```python
from build123d import *

# Parameters (mm, degrees)
EXTRUDE_DEPTH               = 6
EXTRUDE001_DEPTH            = 6
THICKNESS_T                 = 1
BOX002_W                    = 20
BOX002_H                    = 2
BOX002_DEPTH                = 43
BOX_W                       = 5
BOX_H                       = 20
BOX_DEPTH                   = 5
BOX001_W                    = 20
BOX001_H                    = 4
BOX001_DEPTH                = 45
CYLINDER001_W               = 52
CYLINDER001_H               = 50
CYLINDER001_ANGLE           = 60
CYLINDER001_PLACEMENT_ANGLE = 60
CYLINDER_W                  = 54
CYLINDER_H                  = 50
CYLINDER_ANGLE              = 60
CYLINDER_PLACEMENT_ANGLE    = 60


with BuildPart() as extrude_body:
    with BuildSketch(Plane(origin=(8.5, 45, 6), x_dir=(1, 0, 0), z_dir=(0, 1, 0))):
        with BuildLine():
            Line((5, 4), (-5, 4))
            Line((-5, 4), (-5, -3.142136))
            ThreePointArc((-5, -3.142136), (-2.53653, -3.783978), (0, -4))
            ThreePointArc((0, -4), (2.53653, -3.783978), (5, -3.142136))
            Line((5, -3.142136), (5, 4))
        make_face()
    extrude(amount=EXTRUDE_DEPTH)


with BuildPart() as extrude001:
    with BuildSketch(Plane(origin=(8.5, 45, 6), x_dir=(1, 0, 0), z_dir=(0, 1, 0))):
        with BuildLine():
            Line((5, 4), (-5, 4))
            Line((-5, 4), (-5, -3.142136))
            ThreePointArc((-5, -3.142136), (-2.53653, -3.783978), (0, -4))
            ThreePointArc((0, -4), (2.53653, -3.783978), (5, -3.142136))
            Line((5, -3.142136), (5, 4))
        make_face()
    extrude(amount=EXTRUDE001_DEPTH)


with BuildPart() as fusion002:
    # Thickness base: copy of Extrude body
    add(extrude_body.part)

    # Thickness
    thickness_openings = [fusion002.faces().sort_by_distance(p)[0] for p in [
        (8.5, 51, 5.862901),
    ]]
    offset(amount=THICKNESS_T, openings=thickness_openings)

    # Fusion002: union Extrude body, Extrude001
    add(extrude_body.part)
    add(extrude001.part)


with BuildPart() as fusion002_1:
    # Fusion002 placement: moved
    add(fusion002.part.moved(Location((0, -3, 20))))


with BuildPart() as slot:
    # Box002 → Box002 (new body)
    with BuildSketch(Plane(origin=(2, 44, 3.5), x_dir=(1, 0, 0), z_dir=(0, 0, 1))):
        with Locations((10, 1)):
            Rectangle(BOX002_W, BOX002_H)
    extrude(amount=BOX002_DEPTH)


with BuildPart() as pin_opening:
    # Box → Box (new body)
    with BuildSketch(Plane(origin=(7, 42, 5), x_dir=(1, 0, 0), z_dir=(0, 0, 1))):
        with Locations((2.5, 10)):
            Rectangle(BOX_W, BOX_H)
    extrude(amount=BOX_DEPTH)


with BuildPart() as latch:
    # Box001 → Box001 (new body)
    with BuildSketch(Plane(origin=(0, 44, 2.5), x_dir=(1, 0, 0), z_dir=(0, 0, 1))):
        with Locations((10, 2)):
            Rectangle(BOX001_W, BOX001_H)
    extrude(amount=BOX001_DEPTH)


with BuildPart() as bottle_wall001:
    # Cylinder001 → Cylinder001 (revolve)
    with BuildSketch(Plane.XZ):
        with Locations((26, 25)):
            Rectangle(CYLINDER001_W, CYLINDER001_H)
    revolve(axis=Axis((0, 0, 0), (0, 0, 1)), revolution_arc=CYLINDER001_ANGLE)


with BuildPart() as bottle_wall001_1:
    # Cylinder001 placement: moved
    add(bottle_wall001.part.moved(Location((8.5, -7, 0))).rotate(Axis((8.5, -7, 0), (0, 0, 1)), CYLINDER001_PLACEMENT_ANGLE))


with BuildPart() as cut003:
    # Cylinder → Cylinder (revolve)
    with BuildSketch(Plane.XZ):
        with Locations((27, 25)):
            Rectangle(CYLINDER_W, CYLINDER_H)
    revolve(axis=Axis((0, 0, 0), (0, 0, 1)), revolution_arc=CYLINDER_ANGLE)


with BuildPart() as cut003_1:
    # Cylinder placement: moved
    add(cut003.part.moved(Location((8.5, -7, 0))).rotate(Axis((8.5, -7, 0), (0, 0, 1)), CYLINDER_PLACEMENT_ANGLE))

    # Cut: cut bottle_wall001
    add(bottle_wall001_1.part, mode=Mode.SUBTRACT)


with BuildPart() as cut003_2:
    # Cut placement: moved
    add(cut003_1.part.moved(Location((0, -2, 0))))

    # Fusion: union latch
    add(latch.part)

    # Fusion001: union latch
    add(latch.part)

    # Cut001: cut pin_opening
    add(pin_opening.part, mode=Mode.SUBTRACT)

    # Cut002: cut slot
    add(slot.part, mode=Mode.SUBTRACT)

    # Cut003: cut Fusion002
    add(fusion002_1.part, mode=Mode.SUBTRACT)


solid = cut003_2.part
```
Build history of the part. All positions in model axes, mm. A direction names the side the tool comes from. Round coordinates to 2 decimals unless told otherwise and drop trailing zeros. Loops run counter-clockwise (first coordinate to the right, second up) from the corner with the lowest first, then second, coordinate; pieces in that order, holes last.
Item 1: Pin check, flat tips, straight feed: P1, Ø3, axis at y = 46, z = 30, coming from the -X side; P2, Ø8, axis at x = -7, z = 41.5, coming from the -Y side; P3, Ø5, axis at x = -9.5, z = 28.5, coming from the -Y side. Stop position of each tip, or through.
Item 2: Two-plate mould, pull along Y, no slides. Class faces 5 (the face through (11, 45, 46.5)), 6 (the face through (-18, 36.9, 25.4)), 7 (the face through (8, 44, 0)): released by +Y, released by -Y, zero draft, split by the parting line, or undercut.
Item 3: Saw through at C-C (z = 45.5). List the corners of the cut face in (x, y).
Item 4: Saw through at B-B (y = 41.75). List the corners of the cut face in (x, z), then the cut area to 3 significant figures.
Item 5: Saw through at D-D (x = -8.5). List the corners of the cut face in (y, z), then the cut area to 3 significant figures.
Item 6: Which spindle directions (+Z, -Z, +X, -X, +Y, -Y) get a long thin tool onto all of the face, cutting with end or side? Do faces 1 (the face through (2, 45, 25)), 2 (the face through (9, 47, 21)), 3 (the face through (20, 47, 25)), 4 (the face through (0, 46, 25)). Say none if no direction does.
Item 7: Drill centre lines: line 1 along Z through (x, y) = (10.5, 45.5); line 2 along Z through (x, y) = (12, 44.75); line 3 along Y through (x, z) = (2.5, 34). Where is each one in solid material? Low to high.
Item 8: Saw through at A-A (z = 27). List the corners of the cut face in (x, y).
Worked answers:
1. P1: stops at x = 0
1. P2: stops at y = 39.21
1. P3: stops at y = 38.79
2. face 5: undercut
2. face 6: released by -Y
2. face 7: zero draft
3. outline: (-18.5, 37.77) - (-17.5, 36.03) arc R52 cw to (34.5, 36.03) - (35.5, 37.77) arc R54 ccw to (18.84, 44) - (2, 44) - (2, 46) - (20, 46) - (20, 48) - (0, 48) - (0, 44.33) arc R54 ccw to start
4. outline: (-9.95, 0) - (-2.83, 0) - (-2.83, 50) - (-9.95, 50) - close; (19.83, 0) - (26.95, 0) - (26.95, 50) - (19.83, 50) - close
4. area: 712 mm2
5. outline: (40.14, 0) - (42.25, 0) - (42.25, 50) - (40.14, 50) - close
5. area: 106 mm2
6. face 1: +X
6. face 2: +Y, -Y
6. face 3: +Z, -Z, +X, +Y
6. face 4: +Z, -Z, -X, +Y
7. line 1: z = 2.5 to 3.5, 46.5 to 47.5
7. line 2: z = 0 to 3.5, 46.5 to 50
7. line 3: y = 42.65 to 44, 46 to 48
8. outline: (-18.5, 37.77) - (-17.5, 36.03) arc R52 cw to (2.5, 42.65) - (2.5, 44) - (2, 44) - (2, 46) - (2.5, 46) - (2.5, 48) - (0, 48) - (0, 44.33) arc R54 ccw to start; (14.5, 42.65) arc R52 cw to (34.5, 36.03) - (35.5, 37.77) arc R54 ccw to (18.84, 44) - (14.5, 44) - close; (14.5, 46) - (20, 46) - (20, 48) - (14.5, 48) - close
